```python
from build123d import *

# Parameters (mm, degrees)
F0_W      = 479.425
F0_H      = 228.6
F1_DEPTH  = 12.7
F2_R      = 3.175
F3_DEPTH  = 12.701
F4_W      = 479.425
F4_H      = 184.15
F5_DEPTH  = 168.275
F6_W      = 758.825
F6_H      = 158.75
F7_DEPTH  = 25.4
F8_W      = 498.475
F8_H      = 22.225
F9_DEPTH  = 114.3
F10_W     = 127
F10_H     = 22.225
F11_DEPTH = 215.9
F12_SIZE  = 15.875
F14_DEPTH = 15.875


with BuildPart() as f1:
    # F0 (on Top) → F1 (new body)
    with BuildSketch(Plane.XY):
        Rectangle(F0_W, F0_H)
    extrude(amount=F1_DEPTH)

    # F2 (on face) → F3 (cut, through all)
    with BuildSketch(Plane(origin=(0, 0, 0), x_dir=(1, 0, 0), z_dir=(0, 0, -1))):
        with Locations((220.6625, -104.775)):
            Circle(F2_R)
        with Locations((-220.6625, -104.775)):
            Circle(F2_R)
        with Locations((220.6625, 104.775)):
            Circle(F2_R)
        with Locations((-220.6625, 104.775)):
            Circle(F2_R)
    extrude(amount=-F3_DEPTH, mode=Mode.SUBTRACT)

    # F4 (on face) → F5 (join)
    with BuildSketch(Plane.XY.offset(12.7)):
        Rectangle(F4_W, F4_H)
    extrude(amount=F5_DEPTH)

    # F6 (on face) → F7 (join)
    with BuildSketch(Plane.XY.offset(180.975)):
        Rectangle(F6_W, F6_H)
    extrude(amount=F7_DEPTH)

    # F8 (on face) → F9 (join)
    with BuildSketch(Plane.XY.offset(206.375)):
        with Locations((0, -68.2625)):
            Rectangle(F8_W, F8_H)
    extrude(amount=F9_DEPTH)

    # F10 (on face) → F11 (join)
    with BuildSketch(Plane.XZ.offset(79.375)):
        with Locations((0, 192.0875)):
            Rectangle(F10_W, F10_H)
    extrude(amount=F11_DEPTH)

    # F12
    f12_edges = [f1.edges().sort_by_distance(p)[0] for p in [
        (-379.4125, 79.375, 193.675),
        (-379.4125, -79.375, 193.675),
        (379.4125, -79.375, 193.675),
        (379.4125, 79.375, 193.675),
    ]]
    chamfer(f12_edges, length=F12_SIZE)

    # F13 (on face) → F14 (join)
    with BuildSketch(Plane.XY.offset(206.375)):
        with BuildLine():
            ThreePointArc((-76.2, -38.1), (-70.620384, -51.570384), (-57.15, -57.15))
            Line((-57.15, -57.15), (57.15, -57.15))
            ThreePointArc((57.15, -57.15), (70.620384, -51.570384), (76.2, -38.1))
            Line((76.2, -38.1), (76.2, 139.7))
            ThreePointArc((76.2, 139.7), (70.620384, 153.170384), (57.15, 158.75))
            Line((57.15, 158.75), (-57.15, 158.75))
            ThreePointArc((-57.15, 158.75), (-70.620384, 153.170384), (-76.2, 139.7))
            Line((-76.2, 139.7), (-76.2, -38.1))
        make_face()
    extrude(amount=F14_DEPTH)


solid = f1.part
```
The listing builds one solid part. Answer for the finished solid, in the listing's coordinates (mm). A direction names the side the tool comes from. Give positions to 0.01 mm unless a question says otherwise; leave off trailing zeros. Loops run counter-clockwise (first coordinate to the right, second up) from the corner with the lowest first, then second, coordinate; pieces in that order, holes last. Notation, with made-up numbers: (19, 37.5) - (59, 37.5) arc R24 ccw to (59, 60.5) - close; hole circle Ø11 at (59.5, -28.75). An arc over 180 degrees is marked (long way). Return JSON: item names as keys, results as strings. Group by question number.
1. Straight lines are drawn through the part: line 1 (Y direction, x = -85.5, z = 289) (3 decimals); line 2 (Y direction, x = -192, z = 83.5) (3 decimals); line 3 (Z direction, x = -111, y = 43) (3 decimals). For each, find the intervals that lie inside material, in ascending order. Write a range as [from, to].
2. Given pin 1 Ø11 at (y, z) = (-157.5, 190.5) entering from -X; pin 2 Ø18 at (y, z) = (-67.5, 267) entering from +X; pin 3 Ø11 at (x, y) = (12, -108) entering from +Z, each flat-ended and moving along its own axis, determine where each tip first touches the part or whether it passes through.
3. Find section A-A (x = -92). Write down the section's boundary in (y, z) (3 decimals).
4. Find section D-D (x = 11.5). Write down the section's boundary in (y, z) (3 decimals), then the cut area to 3 significant figures.
5. Which of the six approach directions +Z, -Z, +X, -X, +Y, -Y give full straight-line access (tool end or side, diameter ignored) to faces 1 (the flat face through (249.238, -68, 263)), 2 (the flat face through (309, 1, 180.975)), 3 (the flat face through (-3, 92.075, 96))?
Verdict:
{
 "1": {"line 1": "y = [-79.375, -57.15]", "line 2": "y = [-92.075, 92.075]", "line 3": "z = [0, 206.375]"},
 "2": {"pin 1": "stops at x = -63.5", "pin 2": "stops at x = 249.24", "pin 3": "stops at z = 203.2"},
 "3": {"outline": "(-114.3, 0) - (114.3, 0) - (114.3, 12.7) - (92.075, 12.7) - (92.075, 180.975) - (79.375, 180.975) - (79.375, 206.375) - (-57.15, 206.375) - (-57.15, 320.675) - (-79.375, 320.675) - (-79.375, 180.975) - (-92.075, 180.975) - (-92.075, 12.7) - (-114.3, 12.7) - close"},
 "4": {"outline": "(-295.275, 180.975) - (-92.075, 180.975) - (-92.075, 12.7) - (-114.3, 12.7) - (-114.3, 0) - (114.3, 0) - (114.3, 12.7) - (92.075, 12.7) - (92.075, 180.975) - (79.375, 180.975) - (79.375, 206.375) - (158.75, 206.375) - (158.75, 222.25) - (-57.15, 222.25) - (-57.15, 320.675) - (-79.375, 320.675) - (-79.375, 203.2) - (-295.275, 203.2) - close", "area": "48,700 mm^2"},
 "5": {"face 1": "+Z, +X, +Y, -Y", "face 2": "-Z, +X, +Y, -Y", "face 3": "+X, -X, +Y"}
}
